Here's the drawing with two shaded views (mm, measured from the low corner). I have some questions. A direction names the side the tool comes from. Give positions to 0.01 mm unless a question says otherwise; leave off trailing zeros. Loops run counter-clockwise (first coordinate to the right, second up) from the corner with the lowest first, then second, coordinate; pieces in that order, holes last. Notation, with made-up numbers: M 75,55.25 L 126,55.25 A23 cw 126,79.25 Z; hole C -33.5,31.5 d9. An arc over 180 degrees is marked long. Use a Markdown table: item, result. Add a question column.
1) Which directions (+Z, -Z, +X, -X, +Y, -Y) give clear straight access to the entire face, cutting with the end or side of a thin tool? Please do the marked faces 5, 6, 7, 8 and 9.
2) Suppose I cut it at A-A on x = 60.5. List the corners of the cut face in (y, z) for me.
3) Suppose I cut it at D-D on z = 6.5. List the corners of the cut face in (x, y) for me.
4) Suppose I cut it at C-C on x = 18.65. List the corners of the cut face in (y, z) for me, and give its area (3 significant figures).
5) We'd pull the mould along X, two halves only. Please class the marked faces 1, 2, 3 and 4: +X half, -X half, draft (parallel to the pull), parting line (faces both ways), or undercut.
6) If I drill on line 1 along Y through (x, z) = (18.65, 9); line 2 along X through (y, z) = (86, 7.75); line 3 along Y through (x, z) = (61, 13.25), over which ranges is the centre line in solid material (lowest first)? Write a range as [from, to].
7) Will this pin go through, and if not, where does the flat tip stop? pin 1 Ø8 at (y, z) = (35.5, 11) entering from +X.
8) Suppose I cut it at B-B on y = 45.5. List the corners of the cut face in (x, z) for me, and give its area (3 significant figures).
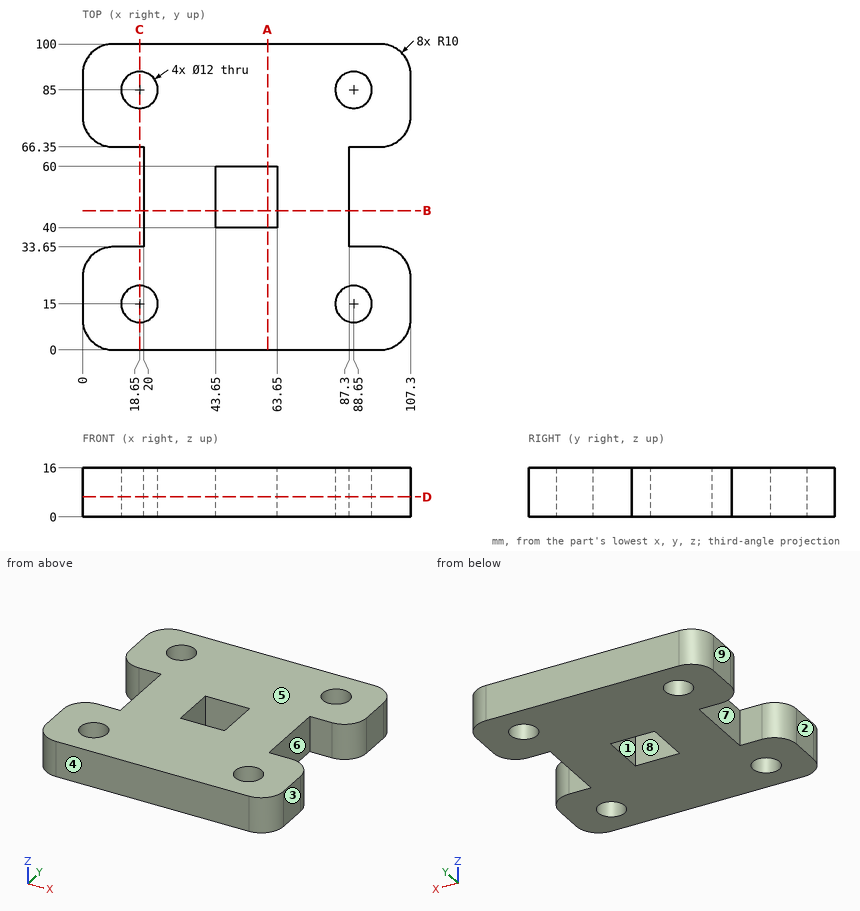
Answer block:
| question | item | result |
|---|---|---|
| 1 | face 5 | +Z, +X, -X, +Y, -Y |
| 1 | face 6 | +Z, -Z, +X |
| 1 | face 7 | +Z, -Z, -X |
| 1 | face 8 | +Z, -Z |
| 1 | face 9 | +Z, -Z, -X, +Y, -Y |
| 2 | outline | M 0,0 L 40,0 L 40,16 L 0,16 Z; M 60,0 L 100,0 L 100,16 L 60,16 Z |
| 3 | outline | M 0,10 A10 ccw 10,0 L 97.3,0 A10 ccw 107.3,10 L 107.3,23.65 A10 ccw 97.3,33.65 L 87.3,33.65 L 87.3,66.35 L 97.3,66.35 A10 ccw 107.3,76.35 L 107.3,90 A10 ccw 97.3,100 L 10,100 A10 ccw 0,90 L 0,76.35 A10 ccw 10,66.35 L 20,66.35 L 20,33.65 L 10,33.65 A10 ccw 0,23.65 Z; hole C 18.65,15 d12; hole C 18.65,85 d12; hole M 43.65,40 L 63.65,40 L 63.65,60 L 43.65,60 Z; hole C 88.65,15 d12; hole C 88.65,85 d12 |
| 4 | outline | M 0,0 L 9,0 L 9,16 L 0,16 Z; M 21,0 L 33.65,0 L 33.65,16 L 21,16 Z; M 66.35,0 L 79,0 L 79,16 L 66.35,16 Z; M 91,0 L 100,0 L 100,16 L 91,16 Z |
| 4 | area | 693 mm^2 |
| 5 | face 1 | undercut |
| 5 | face 2 | -X half |
| 5 | face 3 | +X half |
| 5 | face 4 | draft |
| 6 | line 1 | y = [0, 9], [21, 33.65], [66.35, 79], [91, 100] |
| 6 | line 2 | x = [0, 12.73], [24.57, 82.73], [94.57, 107.3] |
| 6 | line 3 | y = [0, 40], [60, 100] |
| 7 | pin 1 | stops at x = 103.49 |
| 8 | outline | M 20,0 L 43.65,0 L 43.65,16 L 20,16 Z; M 63.65,0 L 87.3,0 L 87.3,16 L 63.65,16 Z |
| 8 | area | 757 mm^2 |
